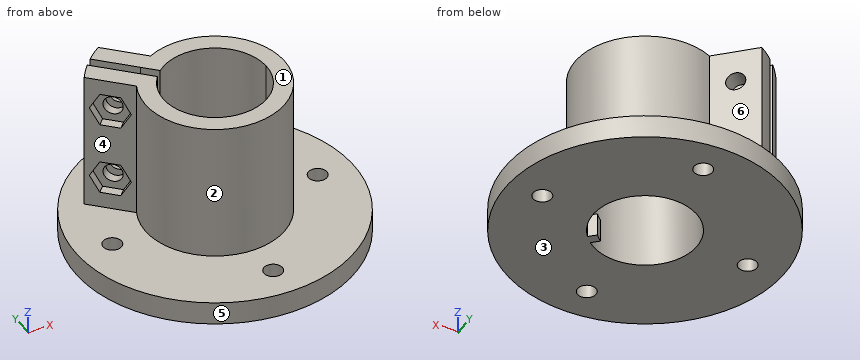
from build123d import *

# Parameters (mm, degrees)
F1_DEPTH = 35
F0_R     = 30
F0_R_2   = 2
F2_DEPTH = 5
F4_R     = 2
F5_DEPTH = 11
F6_DEPTH = 2


with BuildPart() as f1:
    # F0 (on Top) → F1 (new body)
    with BuildSketch(Plane.XY):
        with BuildLine():
            ThreePointArc((-7.1453609838, 8.5595745462), (4.7250251338, 10.0993384677), (11.15, 0))
            ThreePointArc((11.15, 0), (10.4880847772, -3.7845181605), (8.5809277655, -7.119703553))
            ThreePointArc((8.5809277655, -7.119703553), (7.8878989891, -7.880580533), (7.1276656329, -8.5743152861))
            ThreePointArc((7.1276656329, -8.5743152861), (-7.8923790008, -7.8760938103), (-8.5595745462, 7.1453609838))
            Line((-8.5595745462, 7.1453609838), (-11.2901120254, 9.8758984631))
            ThreePointArc((-11.2901120254, 9.8758984631), (-12.5294709258, 8.2469605504), (-13.5355339059, 6.4644660941))
            ThreePointArc((-13.5355339059, 6.4644660941), (10.6066017178, -10.6066017178), (-6.4644660941, 13.5355339059))
            ThreePointArc((-6.4644660941, 13.5355339059), (-8.2469605504, 12.5294709258), (-9.8758984631, 11.2901120254))
            Line((-9.8758984631, 11.2901120254), (-7.1453609838, 8.5595745462))
        make_face()
        with BuildLine():
            ThreePointArc((-13.5355339059, 6.4644660941), (-12.5294709258, 8.2469605504), (-11.2901120254, 9.8758984631))
            Line((-11.2901120254, 9.8758984631), (-18.3706285138, 16.9564149515))
            ThreePointArc((-18.3706285138, 16.9564149515), (-19.6773328655, 15.4208485922), (-20.8560419816, 13.7849741698))
            Line((-20.8560419816, 13.7849741698), (-13.5355339059, 6.4644660941))
        make_face()
        with BuildLine():
            Line((-16.9564149515, 18.3706285138), (-9.8758984631, 11.2901120254))
            ThreePointArc((-9.8758984631, 11.2901120254), (-8.2469605504, 12.5294709258), (-6.4644660941, 13.5355339059))
            Line((-6.4644660941, 13.5355339059), (-13.7849741698, 20.8560419816))
            ThreePointArc((-13.7849741698, 20.8560419816), (-15.4208485922, 19.6773328655), (-16.9564149515, 18.3706285138))
        make_face()
    extrude(amount=F1_DEPTH)

    # F0 (on Top) → F2 (join)
    with BuildSketch(Plane.XY):
        Circle(F0_R)
        with Locations((0, -22.5)):
            Circle(F0_R_2, mode=Mode.SUBTRACT)
        with Locations((-22.5, 0)):
            Circle(F0_R_2, mode=Mode.SUBTRACT)
        with BuildLine():
            Line((-13.7849741698, 20.8560419816), (-6.4644660941, 13.5355339059))
            ThreePointArc((-6.4644660941, 13.5355339059), (10.6066017178, -10.6066017178), (-13.5355339059, 6.4644660941))
            Line((-13.5355339059, 6.4644660941), (-20.8560419816, 13.7849741698))
            ThreePointArc((-20.8560419816, 13.7849741698), (-19.6773328655, 15.4208485922), (-18.3706285138, 16.9564149515))
            ThreePointArc((-18.3706285138, 16.9564149515), (-17.6776695297, 17.6776695297), (-16.9564149515, 18.3706285138))
            ThreePointArc((-16.9564149515, 18.3706285138), (-15.4208485922, 19.6773328655), (-13.7849741698, 20.8560419816))
        make_face(mode=Mode.SUBTRACT)
        with Locations((22.5, 0)):
            Circle(F0_R_2, mode=Mode.SUBTRACT)
        with Locations((0, 22.5)):
            Circle(F0_R_2, mode=Mode.SUBTRACT)
        with BuildLine():
            ThreePointArc((7.1276656329, -8.5743152861), (7.8878989891, -7.880580533), (8.5809277655, -7.119703553))
            Line((8.5809277655, -7.119703553), (7.1560256843, -5.7020870219))
            ThreePointArc((7.1560256843, -5.7020870219), (6.4700270479, -6.4700270479), (5.7020870219, -7.1560256843))
            Line((5.7020870219, -7.1560256843), (7.1276656329, -8.5743152861))
        make_face()
        with BuildLine():
            ThreePointArc((-8.5595745462, 7.1453609838), (-7.8842406102, 7.8842406102), (-7.1453609838, 8.5595745462))
            Line((-7.1453609838, 8.5595745462), (-9.8758984631, 11.2901120254))
            Line((-9.8758984631, 11.2901120254), (-16.9564149515, 18.3706285138))
            ThreePointArc((-16.9564149515, 18.3706285138), (-17.6776695297, 17.6776695297), (-18.3706285138, 16.9564149515))
            Line((-18.3706285138, 16.9564149515), (-11.2901120254, 9.8758984631))
            Line((-11.2901120254, 9.8758984631), (-8.5595745462, 7.1453609838))
        make_face()
    extrude(amount=F2_DEPTH)

    # F4 (on offset) → F5 (cut)
    with BuildSketch(Plane(origin=(-3.5355339059, -3.5355339059, 0), x_dir=(0.7071067812, -0.7071067812, 0), z_dir=(-0.7071067812, -0.7071067812, 0))):
        with Locations((-19.3185165258, 28)):
            Circle(F4_R)
        with Locations((-19.3185165258, 12)):
            Circle(F4_R)
    extrude(amount=-F5_DEPTH, mode=Mode.SUBTRACT)

    # F4 (on offset) → F6 (cut)
    with BuildSketch(Plane(origin=(-3.5355339059, -3.5355339059, 0), x_dir=(0.7071067812, -0.7071067812, 0), z_dir=(-0.7071067812, -0.7071067812, 0))):
        Polygon((-17.2400555567, 31.6), (-21.3969774949, 31.6), (-23.4754384639, 28), (-21.3969774949, 24.4), (-17.2400555567, 24.4), (-15.1615945876, 28), align=None)
        with Locations((-19.3185165258, 28)):
            Circle(F4_R, mode=Mode.SUBTRACT)
        Polygon((-17.2400555567, 15.6), (-21.3969774949, 15.6), (-23.4754384639, 12), (-21.3969774949, 8.4), (-17.2400555567, 8.4), (-15.1615945876, 12), align=None)
        with Locations((-19.3185165258, 12)):
            Circle(F4_R, mode=Mode.SUBTRACT)
    extrude(amount=-F6_DEPTH, mode=Mode.SUBTRACT)


solid = f1.part
Could you check a few things on this model? Use its own coordinates, in mm. Face numbers are marked on the shaded views. A direction names the side the tool comes from. Give positions to 0.01 mm unless a question says otherwise; leave off trailing zeros. Order: outer loops, then holes, each group sorted by start corner. A loop starts at its lowest first (then second) coordinate and runs counter-clockwise, first axis right, second up.
1. Suppose I cut it at C-C (z = 3). List the corners of the cut face in (x, y) for me.
2. Suppose I cut it at A-A (x = 0). List the corners of the cut face in (y, z) for me.
3. I need wall thicknesses on L1, parallel to Y at x = 0, z = 1; L2, parallel to X at y = 9, z = 8.5; L3, parallel to Y at x = -0.5, z = 3. Which ranges of each line are inside material? Lowest first, please.
4. For the marked faces 1 and 2, which set-ups out of +Z, -Z, +X, -X, +Y, -Y let a thin tool reach every point of the face, with its end or its side?
5. Suppose I cut it at B-B (y = -22.5). List the corners of the cut face in (x, z) for me.
6. We'd pull the mould along X, two halves only. Please class the marked faces 3, 4, 5 and 6: pulls with the +X half, pulls with the -X half, needs draft (parallel to the pull), parting line crosses it, or undercut.
7. Will these pins go through, and if not, where does the flat tip stop? P1, Ø4, axis at x = -8.5, z = 10, coming from the +Y side; P2, Ø10, axis at y = 4, z = 24.5, coming from the -X side; P3, Ø5, axis at y = 6.5, z = 27, coming from the +X side.
Solved:
1. outline: circle Ø60 at (0, 0); hole circle Ø4 at (-22.5, 0); hole circle Ø4 at (0, -22.5); hole circle Ø4 at (0, 22.5); hole (5.7, -7.16) arc R9.15 ccw to (7.16, -5.7) - (8.58, -7.12) arc R11.15 ccw (long way) to (7.13, -8.57) - close; hole circle Ø4 at (22.5, 0)
2. outline: (-30, 0) - (-24.5, 0) - (-24.5, 5) - (-30, 5) - close; (-20.5, 0) - (-11.15, 0) - (-11.15, 35) - (-15, 35) - (-15, 5) - (-20.5, 5) - close; (11.15, 0) - (20.5, 0) - (20.5, 5) - (15, 5) - (15, 35) - (11.15, 35) - close; (24.5, 0) - (30, 0) - (30, 5) - (24.5, 5) - close
3. L1: y = -30 to -24.5, -20.5 to -11.15, 11.15 to 20.5, 24.5 to 30
3. L2: x = -15.3 to -10.41, -7.59 to -6.58, 6.58 to 12
3. L3: y = -30 to -24.44, -20.56 to -11.14, 11.14 to 20.56, 24.44 to 30
4. face 1: +Z, +X, -X, +Y, -Y
4. face 2: +Z
5. outline: (-19.84, 0) - (-2, 0) - (-2, 5) - (-19.84, 5) - close; (2, 0) - (19.84, 0) - (19.84, 5) - (2, 5) - close
6. face 3: needs draft
6. face 4: pulls with the -X half
6. face 5: parting line crosses it
6. face 6: undercut
7. P1: stops at y = 17.57
7. P2: stops at x = -16.07
7. P3: stops at x = 14.46
